Source: CAD feature listing. Evaluate the final solid. Frame: model axes, mm. A direction names the side the tool comes from. Round coordinates to 2 decimals unless told otherwise and drop trailing zeros. Order: outer loops, then holes, each group sorted by start corner. A loop starts at its lowest first (then second) coordinate and runs counter-clockwise, first axis right, second up.
```python
from build123d import *

# Parameters (mm, degrees)
SKETCH1_W           = 120
SKETCH1_H           = 80
SKETCH1_R           = 2.2
SKETCH1_R_2         = 11.1
BOSS_EXTRUDE1_DEPTH = 2


with BuildPart() as part:
    # Sketch1 → Boss-Extrude1 (new body)
    with BuildSketch(Plane(origin=(0, 0, 0), x_dir=(1, 0, 0), z_dir=(0, 1, 0))):
        Rectangle(SKETCH1_W, SKETCH1_H)
        with Locations(Location((-52.5, 35, 0), (0, 0, 270))):
            Circle(SKETCH1_R, mode=Mode.SUBTRACT)
        with Locations(Location((52.5, 35, 0), (0, 0, 90))):
            Circle(SKETCH1_R, mode=Mode.SUBTRACT)
        with Locations(Location((52.5, -35, 0), (0, 0, 270))):
            Circle(SKETCH1_R, mode=Mode.SUBTRACT)
        with Locations(Location((-52.5, -35, 0), (0, 0, 90))):
            Circle(SKETCH1_R, mode=Mode.SUBTRACT)
        with Locations(Location((0, 0, 0), (0, 0, 270))):
            Circle(SKETCH1_R_2, mode=Mode.SUBTRACT)
        with BuildLine():
            Line((-17.7, -30), (-17.7, 30))
            ThreePointArc((-17.7, 30), (-15.5, 32.2), (-13.3, 30))
            Line((-13.3, 30), (-13.3, -30))
            ThreePointArc((-13.3, -30), (-15.5, -32.2), (-17.7, -30))
        make_face(mode=Mode.SUBTRACT)
        with BuildLine():
            Line((13.3, 30), (13.3, -30))
            ThreePointArc((13.3, -30), (15.5, -32.2), (17.7, -30))
            Line((17.7, -30), (17.7, 30))
            ThreePointArc((17.7, 30), (15.5, 32.2), (13.3, 30))
        make_face(mode=Mode.SUBTRACT)
    extrude(amount=BOSS_EXTRUDE1_DEPTH)


solid = part.part
```
1. Line query: line 1 along X through (y, z) = (0.45, 0); line 2 along X through (y, z) = (0.3, -22); line 3 along X through (y, z) = (0.75, 35). Output: solid intervals per line, ascending.
2. Section C-C on x = -52.5. Return loops of the section in (y, z).
3. Pull-direction query (Z, two-part tool) for faces 1 (the face through (12, 0, -1)), 2 (the face through (15.5, 1, -32.2)); classes: released by +Z, released by -Z, zero draft, split by the parting line, or undercut.
4. Section B-B on z = 18. Return loops of the section in (x, y).
5. Section D-D on y = 0.75. Return loops of the section in (x, z), plus the area to 3 significant figures.
6. Section A-A on x = -15.5. Return loops of the section in (y, z).
7. Access query for faces 3 (the face through (12, 2, -1)), 4 (the face through (15.5, 1, 32.2)). Directions: +Z, -Z, +X, -X, +Y, -Y. A direction counts if a zero-diameter tool reaches every point of the face in a straight line with its end or side. Return the directions, or none.
Result:
1. line 1: x = -60 to -17.7, -13.3 to -11.1, 11.1 to 13.3, 17.7 to 60
1. line 2: x = -60 to -17.7, -13.3 to 13.3, 17.7 to 60
1. line 3: x = -60 to -54.7, -50.3 to 50.3, 54.7 to 60
2. outline: (0, -40) - (2, -40) - (2, -37.2) - (0, -37.2) - close; (0, -32.8) - (2, -32.8) - (2, 32.8) - (0, 32.8) - close; (0, 37.2) - (2, 37.2) - (2, 40) - (0, 40) - close
3. face 1: zero draft
3. face 2: undercut
4. outline: (-60, 0) - (-17.7, 0) - (-17.7, 2) - (-60, 2) - close; (-13.3, 0) - (13.3, 0) - (13.3, 2) - (-13.3, 2) - close; (17.7, 0) - (60, 0) - (60, 2) - (17.7, 2) - close
5. outline: (-60, -40) - (60, -40) - (60, 40) - (-60, 40) - close; hole circle Ø4.4 at (-52.5, -35); hole circle Ø4.4 at (-52.5, 35); hole (-17.7, -30) arc R2.2 ccw to (-13.3, -30) - (-13.3, 30) arc R2.2 ccw to (-17.7, 30) - close; hole circle Ø22.2 at (0, 0); hole (13.3, -30) arc R2.2 ccw to (17.7, -30) - (17.7, 30) arc R2.2 ccw to (13.3, 30) - close; hole circle Ø4.4 at (52.5, -35); hole circle Ø4.4 at (52.5, 35)
5. area: 8,590 mm2
6. outline: (0, -40) - (2, -40) - (2, -32.2) - (0, -32.2) - close; (0, 32.2) - (2, 32.2) - (2, 40) - (0, 40) - close
7. face 3: +Z, -Z, +X, -X, +Y
7. face 4: +Y, -Y
